For this review, take the finished solid that the model builds, in its own axes (mm). A direction names the side the tool comes from. Give positions to 0.01 mm unless a question says otherwise; leave off trailing zeros. Order: outer loops, then holes, each group sorted by start corner. A loop starts at its lowest first (then second) coordinate and runs counter-clockwise, first axis right, second up. Notation, with made-up numbers: (54, 23.5) - (85, 23.5) arc R10 cw to (85, 36.5) - close; hole circle Ø2 at (80.5, -32.5). An arc over 180 degrees is marked (long way). One line per item, written item: value.
```python
from build123d import *

# Parameters (mm, degrees)
F0_R      = 13.5
F1_DEPTH  = 0.6
F2_R      = 0.59999
F5_R      = 10.9
F6_DEPTH  = 8.9
F9_DEPTH  = 7
F10_DEPTH = 7
F11_DEPTH = 25
F12_DEPTH = 7
F14_DEPTH = 3


# Not quite as in the source:
# - a fillet or chamfer is up to 0.001 mm smaller than in the source, because OpenCascade refuses the exact size


with BuildPart() as f1:
    # F0 (on Top) → F1 (new body)
    with BuildSketch(Plane.XY):
        Circle(F0_R)
    extrude(amount=F1_DEPTH)

    # F2 (radius 0.6 in the source; OpenCascade refuses exactly that, so slightly less here)
    f2_edges = [f1.edges().sort_by_distance(p)[0] for p in [
        (-13.5, 0, 0),
    ]]
    fillet(f2_edges, radius=F2_R)

    # F5 (on face) → F6 (join)
    with BuildSketch(Plane.XY.offset(0.6)):
        Circle(F5_R)
    extrude(amount=F6_DEPTH)

    # F3 (on Front) → F9 (cut)
    with BuildSketch(Plane.XZ):
        Polygon((-0.5, 0), (0, 0), (0.5, 0), (0.5, 1), (1.5, 1), (1.5, 0), (2.5, 0), (2.5, 1), (3.5, 1), (3.5, 0), (4.5, 0), (4.5, 4.2), (-4.5, 4.2), (-4.5, 0), (-3.5, 0), (-3.5, 1), (-2.5, 1), (-2.5, 0), (-1.5, 0), (-1.5, 1), (-0.5, 1), align=None)
    extrude(amount=-F9_DEPTH, mode=Mode.SUBTRACT)

    # F4 (on Front) → F10 (cut)
    with BuildSketch(Plane.XZ):
        Polygon((-0.5, 0), (0, 0), (0.5, 0), (0.5, 1), (1.5, 1), (1.5, 0), (2.5, 0), (2.5, 1), (3.5, 1), (3.5, 0), (4.5, 0), (4.5, 4.2), (-4.5, 4.2), (-4.5, 0), (-3.5, 0), (-3.5, 1), (-2.5, 1), (-2.5, 0), (-1.5, 0), (-1.5, 1), (-0.5, 1), align=None)
    extrude(amount=F10_DEPTH, mode=Mode.SUBTRACT)

    # F7 (on Front) → F11 (cut)
    with BuildSketch(Plane.XZ):
        Polygon((-7.75, 4.2), (0, 4.2), (7.75, 4.2), (7.75, 9.5), (-7.75, 9.5), align=None)
    extrude(amount=-F11_DEPTH, mode=Mode.SUBTRACT)

    # F8 (on Front) → F12 (cut)
    with BuildSketch(Plane.XZ):
        Polygon((-7.75, 4.2), (0, 4.2), (7.75, 4.2), (7.75, 9.5), (-7.75, 9.5), align=None)
    extrude(amount=F12_DEPTH, mode=Mode.SUBTRACT)

    # F13 (on face) → F14 (cut)
    with BuildSketch(Plane.XY.offset(9.5)):
        with BuildLine():
            Line((-7.75, -2.5), (-7.75, 0))
            Line((-7.75, 0), (-7.75, 2.5))
            Line((-7.75, 2.5), (-10.6094297679, 2.5))
            ThreePointArc((-10.6094297679, 2.5), (-10.9, 0), (-10.6094297679, -2.5))
            Line((-10.6094297679, -2.5), (-7.75, -2.5))
        make_face()
        with BuildLine():
            Line((7.75, 2.5), (7.75, 0))
            Line((7.75, 0), (7.75, -2.5))
            Line((7.75, -2.5), (10.6094297679, -2.5))
            ThreePointArc((10.6094297679, -2.5), (10.8271137537, -1.2584147826), (10.9, 0))
            ThreePointArc((10.9, 0), (10.8271137537, 1.2584147826), (10.6094297679, 2.5))
            Line((10.6094297679, 2.5), (7.75, 2.5))
        make_face()
    extrude(amount=-F14_DEPTH, mode=Mode.SUBTRACT)


solid = f1.part
```
(1) Draft analysis for pull direction X (two halves, no side actions). For faces 4 (the face through (-9, -2.5, 8)), 5 (the face through (-0.5, 0.1, 0.5)), 6 (the face through (-2.36, -10.64, 4.99)), state which applies: pulls with the +X half, pulls with the -X half, needs draft (parallel to the pull), parting line crosses it, or undercut.
Answers below:
face 4: needs draft
face 5: undercut
face 6: parting line crosses it
(2) Take a section at D-D (z = 1.75). Write out the cut boundary in (x, y).
Answers below:
outline: circle Ø21.8 at (0, 0); hole (-4.5, -7) - (4.5, -7) - (4.5, 7) - (-4.5, 7) - close
(3) Wall thickness on line 1 (Y direction, x = -1.25, z = 3); line 2 (Z direction, x = 11.25, y = 2.75); line 3 (Y direction, x = -1, z = 1.25): over which ranges is each line inside the solid? List them lowest first. Write a range as from..to.
Answers below:
line 1: y = -10.83..-7, 7..10.83
line 2: z = 0..0.6
line 3: y = -10.85..-7, 7..10.85
(4) For P1, Ø1, axis at x = -7.5, y = 9, coming from the -Z side; P2, Ø1, axis at x = 6.5, z = 7.5, coming from the +Y side; P3, Ø3, axis at x = 3, z = 3.5, coming from the +Y side; P4, Ø0.5, axis at x = 1, y = 1.5, coming from the +Z side, all flat-tipped, find the tip position at first contact; note any pin that passes through.
Answers below:
P1: stops at z = 0
P2: stops at y = -7
P3: stops at y = 10.8
P4: stops at z = 1
(5) Take a section at A-A (z = 7.5). Write out the cut boundary in (x, y).
Answers below:
outline: (-10.61, -2.5) arc R10.9 ccw to (10.61, -2.5) - (7.75, -2.5) - (7.75, -7) - (-7.75, -7) - (-7.75, -2.5) - close; (-10.61, 2.5) - (-7.75, 2.5) - (-7.75, 7.66) arc R10.9 ccw to start; (7.75, 2.5) - (10.61, 2.5) arc R10.9 ccw to (7.75, 7.66) - close
(6) Take a section at B-B (y = 0). Give the number of separate pieces and of enclosed holes in the cut face, then the cut area to 3 significant figures.
Answers below:
separate pieces: 6
enclosed holes: 0
area: 75.2 mm^2
(7) Machinability: for faces 1 (the face through (7.75, 0, 6)), 2 (the face through (0, 7, 2)), 3 (the face through (4.5, 0, 2)), which of the approach directions +Z, -Z, +X, -X, +Y, -Y give a long, thin tool a straight path to every point of the face, cutting with its end or side? Answer none if there is none.
Answers below:
face 1: +Z, +Y
face 2: +Z
face 3: +Z, -Z
